Source: CAD feature listing. Evaluate the final solid. Frame: model axes, mm. Face numbers are marked on the shaded views. Coordinates: 2 decimals unless noted, no trailing zeros. Loops run counter-clockwise (first coordinate to the right, second up) from the corner with the lowest first, then second, coordinate; pieces in that order, holes last.
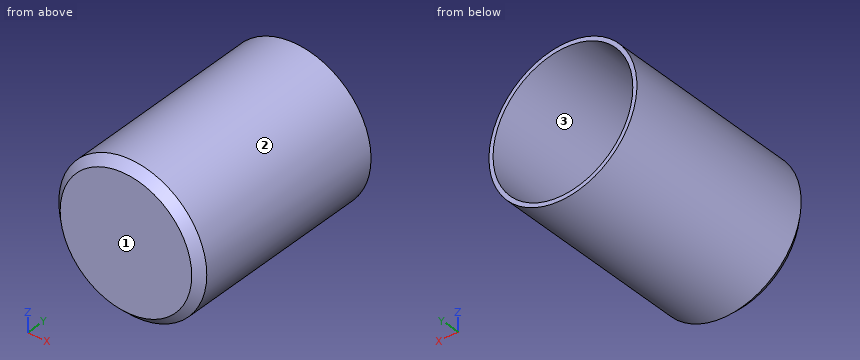
from build123d import *

# Parameters (mm, degrees)
F0_R     = 45.877581
F1_DEPTH = 127
F2_SIZE  = 5.08
F3_T     = -2.54


with BuildPart() as f1:
    # F0 (on Front) → F1 (new body)
    with BuildSketch(Plane.XZ):
        Circle(F0_R)
    extrude(amount=F1_DEPTH)

    # F2
    f2_edges = [f1.edges().sort_by_distance(p)[0] for p in [
        (-45.877581, -127, 0),
    ]]
    chamfer(f2_edges, length=F2_SIZE)

    # F3
    f3_openings = [f1.faces().sort_by_distance(p)[0] for p in [
        (0, 0, 0),
    ]]
    offset(amount=F3_T, openings=f3_openings)


solid = f1.part
Q1. Line query: line 1 along Y through (x, z) = (-20, 8); line 2 along Z through (x, y) = (-34, -6.5); line 3 along Z through (x, y) = (0, -36.5). Output: solid intervals per line, ascending.
Q2. Section C-C, the plane y = -43. Return the cut outline in (x, z), plus the area to 3 significant figures.
Q3. Section B-B, the plane z = 0. Return the cut outline in (x, y), plus the area to 3 significant figures.
Q4. Draft query along Z for the marked faces 1, 2 and 3. Return one class per face: +Z half, -Z half, draft (parallel to the pull), parting line (faces both ways), or undercut.
Q5. Contact query for flat-ended pins moving along their axis: pin 1 Ø1 at (y, z) = (-41, -3) entering from -X; pin 2 Ø24 at (x, z) = (14.5, 19) entering from +Y; pin 3 Ø5 at (x, z) = (-36.5, -9) entering from +Y. Output: stop coordinate, or through.
Q6. Section A-A, the plane x = 0. Return the cut outline in (y, z), plus the area to 3 significant figures.
Derived:
1. line 1: y = -127 to -124.46
1. line 2: z = -30.8 to -26.87, 26.87 to 30.8
1. line 3: z = -45.88 to -43.34, 43.34 to 45.88
2. outline: circle Ø91.76 at (0, 0); hole circle Ø86.68 at (0, 0)
2. area: 712 mm2
3. outline: (-45.88, -121.92) - (-40.8, -127) - (40.8, -127) - (45.88, -121.92) - (45.88, 0) - (43.34, 0) - (43.34, -120.87) - (39.75, -124.46) - (-39.75, -124.46) - (-43.34, -120.87) - (-43.34, 0) - (-45.88, 0) - close
3. area: 852 mm2
4. face 1: draft
4. face 2: parting line
4. face 3: undercut
5. pin 1: stops at x = -45.81
5. pin 2: stops at y = -124.46
5. pin 3: stops at y = -124.11
6. outline: (-127, -40.8) - (-121.92, -45.88) - (0, -45.88) - (0, -43.34) - (-120.87, -43.34) - (-124.46, -39.75) - (-124.46, 39.75) - (-120.87, 43.34) - (0, 43.34) - (0, 45.88) - (-121.92, 45.88) - (-127, 40.8) - close
6. area: 852 mm2
